Can you work these out from the model? Positions are in its coordinate system, mm. Face numbers are marked on the shaded views. Round coordinates to 2 decimals unless told otherwise and drop trailing zeros. Write each loop counter-clockwise with the first axis right and the second up, starting at its lowest first coordinate (ties: lowest second). Pieces come first, ordered by that corner, then holes. Notation, with made-up numbers: (-0.75, 37) - (35.25, 37) arc R35 ccw to (35.25, 71) - close; hole circle Ø10 at (-16, -21.75). An arc over 180 degrees is marked (long way). One line per item, written item: value. Start each with the question number.
(1) If I drill on L1, parallel to Z at x = 2.7, y = 0 (3 decimals); L2, parallel to Z at x = 0.8, y = 0.75, over which ranges is the centre line in solid material (lowest first)? Write a range as from..to.
(2) I'm going to push flat-ended pins straight in: pin 1 Ø5 at (y, z) = (-3.5, 4) entering from -X; pin 2 Ø2 at (x, y) = (2.5, -3.5) entering from +Z; pin 3 Ø1.5 at (x, y) = (2.5, -3) entering from +Z; pin 4 Ø2 at (x, y) = (2, -4.5) entering from -Z. Where does each tip first touch, or does it pass through?
(3) Thinking about a two-plate mould opening in Y: for the marked faces 1, 2 and 3, which applies, +Y half, -Y half, draft (parallel to the pull), parting line (faces both ways), or undercut?
(4) I want a section at A-A on y = 0. List the corners of the cut face in (x, z) for me (3 decimals).
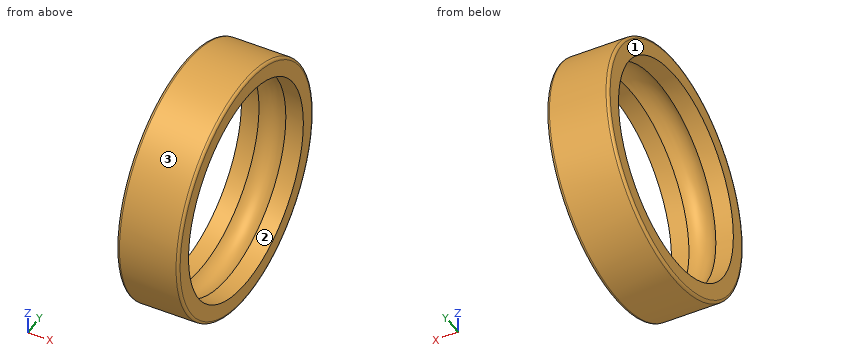
from build123d import *


with BuildPart() as part:
    # Sketch1 → Revolve1 (revolve)
    with BuildSketch(Plane.XY):
        with BuildLine():
            Line((0, 6.85), (0, 5.975))
            Line((0, 5.975), (0.990477123, 5.975))
            ThreePointArc((0.990477123, 5.975), (1.75, 6.3), (2.509522877, 5.975))
            Line((2.509522877, 5.975), (3.5, 5.975))
            Line((3.5, 5.975), (3.5, 6.85))
            ThreePointArc((3.5, 6.85), (3.456066017, 6.956066017), (3.35, 7))
            Line((3.35, 7), (0.15, 7))
            ThreePointArc((0.15, 7), (0.043933983, 6.956066017), (0, 6.85))
        make_face()
    revolve(axis=Axis((3.5, 0, 0), (-1, 0, 0)))


solid = part.part
Established:
1. L1: -7..-5.975, 5.975..7
1. L2: -6.96..-5.93, 5.93..6.96
2. pin 1: x = 0
2. pin 2: z = 6.54
2. pin 3: z = 6.63
2. pin 4: z = -6.06
3. face 1: draft
3. face 2: undercut
3. face 3: parting line
4. outline: (0, -6.85) arc R0.15 ccw to (0.15, -7) - (3.35, -7) arc R0.15 ccw to (3.5, -6.85) - (3.5, -5.975) - (2.51, -5.975) arc R1.05 cw to (0.99, -5.975) - (0, -5.975) - close; (0, 5.975) - (0.99, 5.975) arc R1.05 cw to (2.51, 5.975) - (3.5, 5.975) - (3.5, 6.85) arc R0.15 ccw to (3.35, 7) - (0.15, 7) arc R0.15 ccw to (0, 6.85) - close
